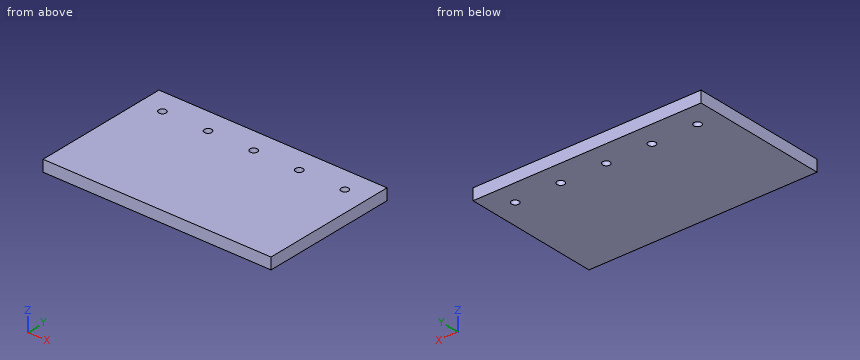
Autodesk Inventor part; units mm, degrees
ref_plane "YZ Plane" through (0, 0, 0) normal (1, 0, 0) x (0, 1, 0)
ref_plane "XZ Plane" through (0, 0, 0) normal (0, 1, 0) x (-1, 0, 0)
ref_plane "XY Plane" through (0, 0, 0) normal (0, 0, 1) x (1, 0, 0)
sketch "Sketch1" plane through (0, 0, 0) normal (0, 0, 1) x (1, 0, 0)
  line L0 (-63.5, -38.1) -> (63.5, -38.1)
  line L1 (63.5, -38.1) -> (63.5, 38.1)
  line L2 (63.5, 38.1) -> (-63.5, 38.1)
  line L3 (-63.5, 38.1) -> (-63.5, -38.1)
  line L4 (-63.5, -38.1) -> (63.5, 38.1) construction
  line L5 (63.5, -38.1) -> (-63.5, 38.1) construction
  point P0 (0, 0)
  dimension "d0" = 127
  dimension "d1" = 76.2
extrude "Extrusion1" add sketch "Sketch1" along normal mid plane 6.35
sketch "Sketch2" plane through (0, 0, 3.175) normal (0, 0, 1) x (1, 0, 0)
  line L0 (-63.5, 38.1) -> (-63.5, -38.1)
  line L1 (63.5, 38.1) -> (-63.5, 38.1)
  point P0 (0, 0)
  point P1 (-50.8, 25.4)
  point P2 (-25.4, 25.4)
  point P3 (0, 25.4)
  point P4 (25.4, 25.4)
  point P5 (50.8, 25.4)
  dimension "d4" = 25.4
  dimension "d5" = 25.4
  dimension "d6" = 25.4
  dimension "d8" = 12.7
  dimension "d9" = 12.7
  dimension "d17" = 25.4
hole "Hole2" at (-50.8, 25.4, 3.175) at (-25.4, 25.4, 3.175) at (0, 25.4, 3.175) at (25.4, 25.4, 3.175) at (50.8, 25.4, 3.175) direction (0, 0, -1) diameter 4.1402 end through all
properties part number "Extender_pulley_gusset"
Could you check a few things on this model? Use its own coordinates, in mm. Round coordinates to 2 decimals unless told otherwise and drop trailing zeros. Order: outer loops, then holes, each group sorted by start corner. A loop starts at its lowest first (then second) coordinate and runs counter-clockwise, first axis right, second up.
(1) I'm going to push a flat-ended pin straight in: pin 1 (3.5 mm diameter, centred on x = 50.8, y = 25.4, fed in from +Z). Where does the tip first touch, or does it pass through?
Response values:
pin 1: passes through
(2) Please list where these lines run through material, in increasing order: line 1 along X through (y, z) = (25.4, -0.75); line 2 along Y through (x, z) = (-25.4, -0.75); line 3 along Y through (x, z) = (-26.5, -1.75).
Response values:
line 1: x = -63.5 to -52.87, -48.73 to -27.47, -23.33 to -2.07, 2.07 to 23.33, 27.47 to 48.73, 52.87 to 63.5
line 2: y = -38.1 to 23.33, 27.47 to 38.1
line 3: y = -38.1 to 23.65, 27.15 to 38.1
(3) Imagine slicing it at B-B (y = 25.4). Write out the boundary of the cut face in (x, z) (3 decimals), plus the area to 3 significant figures.
Response values:
outline: (-63.5, -3.175) - (-52.87, -3.175) - (-52.87, 3.175) - (-63.5, 3.175) - close; (-48.73, -3.175) - (-27.47, -3.175) - (-27.47, 3.175) - (-48.73, 3.175) - close; (-23.33, -3.175) - (-2.07, -3.175) - (-2.07, 3.175) - (-23.33, 3.175) - close; (2.07, -3.175) - (23.33, -3.175) - (23.33, 3.175) - (2.07, 3.175) - close; (27.47, -3.175) - (48.73, -3.175) - (48.73, 3.175) - (27.47, 3.175) - close; (52.87, -3.175) - (63.5, -3.175) - (63.5, 3.175) - (52.87, 3.175) - close
area: 675 mm2
(4) Imagine slicing it at A-A (x = 0). Write out the boundary of the cut face in (y, z) (3 decimals).
Response values:
outline: (-38.1, -3.175) - (23.33, -3.175) - (23.33, 3.175) - (-38.1, 3.175) - close; (27.47, -3.175) - (38.1, -3.175) - (38.1, 3.175) - (27.47, 3.175) - close
